Work out the finished part from the listing and answer in its coordinate system (mm). A direction names the side the tool comes from. Round coordinates to 2 decimals unless told otherwise and drop trailing zeros. Order: outer loops, then holes, each group sorted by start corner. A loop starts at its lowest first (then second) coordinate and runs counter-clockwise, first axis right, second up. Notation, with made-up numbers: (-22, -8.5) - (32, -8.5) arc R24 ccw to (32, 14.5) - close; hole circle Ø8 at (-9.75, -23). An arc over 180 degrees is marked (long way). Use one line per item in the form item = value. Start each with the question number.
Q1. Given P1, Ø0.5, axis at x = 3.5, z = 0.5, coming from the +Y side, flat-ended and moving along its own axis, determine where the tip first touches the part or whether it passes through.
Q2. The part is cut by section C-C on z = 3. Determine the outline of the cut face in (x, y).
Q3. Which of the six approach directions +Z, -Z, +X, -X, +Y, -Y give full straight-line access (tool end or side, diameter ignored) to faces 4 (the flat face through (12.7, 3, 0)), 5 (the flat face through (-6, 6.05, 0))?
Q4. The part is cut by section D-D on x = 10. Determine the outline of the cut face in (y, z).
Q5. The part is cut by section B-B on x = 6.35. Determine the outline of the cut face in (y, z) (3 decimals).
Q6. The part is cut by section A-A on y = -1.5. State how many separate pieces and enclosed holes the cut face has, plus the area to 3 significant figures.
Q7. For a pull along X with two mould halves and no side action, classify faces 1 (the flat face through (0, 6.1, 0)), 2 (the flat face through (4, 6.05, 0)), 3 (the flat face through (-12.7, 3, 0)) as +X half, -X half, draft (parallel to the pull), parting line (faces both ways), or undercut.
Q8. Find the intervals of material crossed by line 1 (Y direction, x = -9, z = -0.25); line 2 (Y direction, x = -10.25, z = -1.75), in increasing order. Write a range as [from, to].
from build123d import *

# Parameters (mm, degrees)
SKETCH1_W           = 25.4
SKETCH1_H           = 10.16
BOSS_EXTRUDE1_DEPTH = 6.1
SKETCH2_W           = 1.52
SKETCH2_H           = 5.08
CUT_EXTRUDE1_DEPTH  = 0.05
SKETCH3_R           = 0.305
BOSS_EXTRUDE2_DEPTH = 4.06
SKETCH4_R           = 0.25
CUT_EXTRUDE2_DEPTH  = 0.1


with BuildPart() as part:
    # Sketch1 → Boss-Extrude1 (new body)
    with BuildSketch(Plane(origin=(0, 0, 0), x_dir=(1, 0, 0), z_dir=(0, 1, 0))):
        Rectangle(SKETCH1_W, SKETCH1_H)
    extrude(amount=BOSS_EXTRUDE1_DEPTH)

    # Sketch2 → Cut-Extrude1 (cut)
    with BuildSketch(Plane(origin=(0, 6.1, 0), x_dir=(1, 0, 0), z_dir=(0, 1, 0))):
        with Locations((-3.81, 0)):
            Rectangle(SKETCH2_W, SKETCH2_H)
        with Locations((-1.27, 0)):
            Rectangle(SKETCH2_W, SKETCH2_H)
        with Locations((-6.35, 0)):
            Rectangle(SKETCH2_W, SKETCH2_H)
        with Locations((-8.89, 0)):
            Rectangle(SKETCH2_W, SKETCH2_H)
        with Locations((-11.43, 0)):
            Rectangle(SKETCH2_W, SKETCH2_H)
        with Locations((11.43, 0)):
            Rectangle(SKETCH2_W, SKETCH2_H)
        with Locations((8.89, 0)):
            Rectangle(SKETCH2_W, SKETCH2_H)
        with Locations((6.35, 0)):
            Rectangle(SKETCH2_W, SKETCH2_H)
        with Locations((3.81, 0)):
            Rectangle(SKETCH2_W, SKETCH2_H)
        with Locations((1.27, 0)):
            Rectangle(SKETCH2_W, SKETCH2_H)
    extrude(amount=-CUT_EXTRUDE1_DEPTH, mode=Mode.SUBTRACT)

    # Sketch3 → Boss-Extrude2 (add)
    with BuildSketch(Plane.XZ):
        with Locations(Location((-1.27, 3.81, 0), (0, 0, 270))):
            Circle(SKETCH3_R)
        with Locations(Location((-3.81, 3.81, 0), (0, 0, 270))):
            Circle(SKETCH3_R)
        with Locations(Location((-6.35, 3.81, 0), (0, 0, 270))):
            Circle(SKETCH3_R)
        with Locations(Location((-8.89, 3.81, 0), (0, 0, 270))):
            Circle(SKETCH3_R)
        with Locations(Location((-11.43, 3.81, 0), (0, 0, 270))):
            Circle(SKETCH3_R)
        with Locations(Location((-3.81, -3.81, 0), (0, 0, 270))):
            Circle(SKETCH3_R)
        with Locations(Location((-6.35, -3.81, 0), (0, 0, 270))):
            Circle(SKETCH3_R)
        with Locations(Location((-8.89, -3.81, 0), (0, 0, 270))):
            Circle(SKETCH3_R)
        with Locations(Location((-11.43, -3.81, 0), (0, 0, 270))):
            Circle(SKETCH3_R)
        with Locations(Location((-1.27, -3.81, 0), (0, 0, 270))):
            Circle(SKETCH3_R)
        with Locations(Location((11.43, -3.81, 0), (0, 0, 90))):
            Circle(SKETCH3_R)
        with Locations(Location((8.89, -3.81, 0), (0, 0, 90))):
            Circle(SKETCH3_R)
        with Locations(Location((6.35, -3.81, 0), (0, 0, 90))):
            Circle(SKETCH3_R)
        with Locations(Location((3.81, -3.81, 0), (0, 0, 90))):
            Circle(SKETCH3_R)
        with Locations(Location((1.27, -3.81, 0), (0, 0, 90))):
            Circle(SKETCH3_R)
        with Locations(Location((1.27, 3.81, 0), (0, 0, 90))):
            Circle(SKETCH3_R)
        with Locations(Location((3.81, 3.81, 0), (0, 0, 90))):
            Circle(SKETCH3_R)
        with Locations(Location((6.35, 3.81, 0), (0, 0, 90))):
            Circle(SKETCH3_R)
        with Locations(Location((8.89, 3.81, 0), (0, 0, 90))):
            Circle(SKETCH3_R)
        with Locations(Location((11.43, 3.81, 0), (0, 0, 90))):
            Circle(SKETCH3_R)
    extrude(amount=BOSS_EXTRUDE2_DEPTH)

    # Sketch4 → Cut-Extrude2 (cut)
    with BuildSketch(Plane.XY.offset(5.08)):
        with Locations((-11.43, 0.790183666)):
            Circle(SKETCH4_R)
    extrude(amount=-CUT_EXTRUDE2_DEPTH, mode=Mode.SUBTRACT)


solid = part.part
Found:
q1.P1 = 6.05
q2.outline = (-12.7, 0) - (12.7, 0) - (12.7, 6.1) - (-12.7, 6.1) - close
q3.face_4 = +Z, -Z, +X, +Y, -Y
q3.face_5 = +Y
q4.outline = (0, -5.08) - (6.1, -5.08) - (6.1, 5.08) - (0, 5.08) - close
q5.outline = (-4.06, -4.115) - (0, -4.115) - (0, -5.08) - (6.1, -5.08) - (6.1, -2.54) - (6.05, -2.54) - (6.05, 2.54) - (6.1, 2.54) - (6.1, 5.08) - (0, 5.08) - (0, 4.115) - (-4.06, 4.115) - (-4.06, 3.505) - (0, 3.505) - (0, -3.505) - (-4.06, -3.505) - close
q6.separate_pieces = 20
q6.enclosed_holes = 0
q6.area = 5.84 mm²
q7.face_1 = draft
q7.face_2 = undercut
q7.face_3 = -X half
q8.line_1 = [0, 6.05]
q8.line_2 = [0, 6.1]
